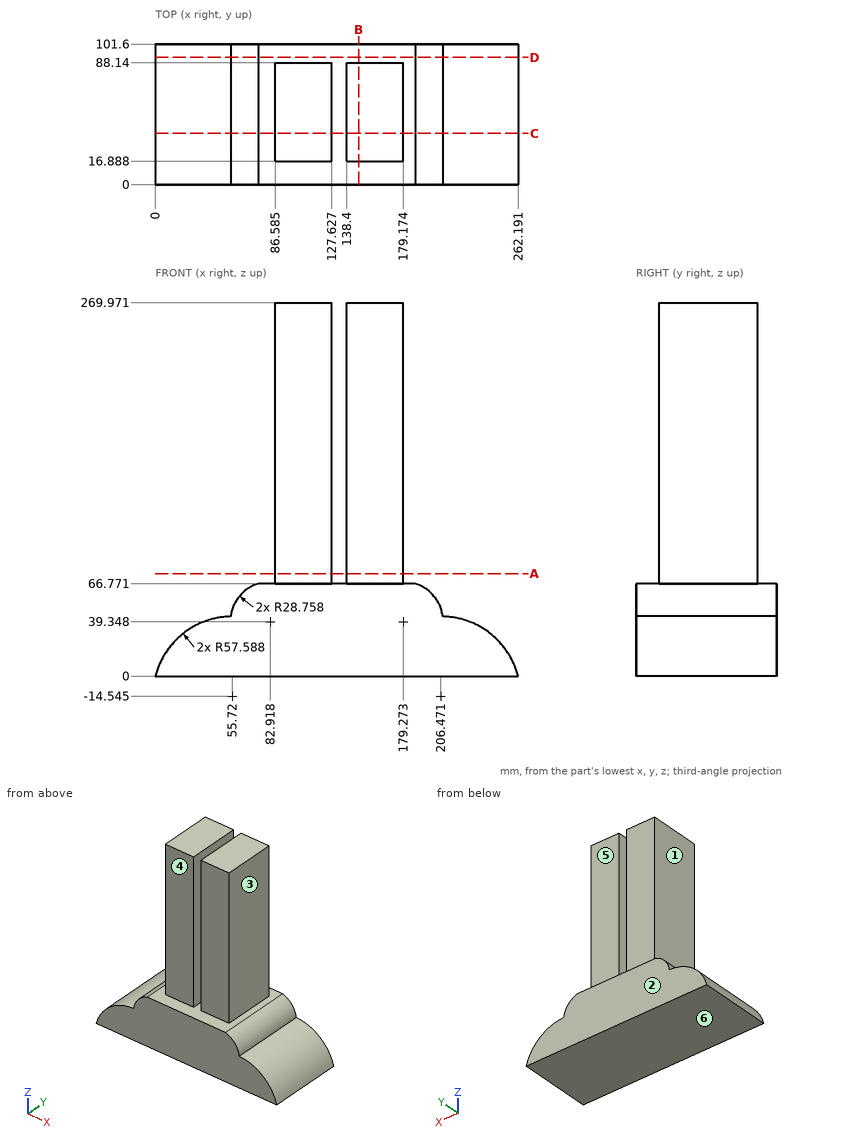
Can you work these out from the drawing? Everything is in mm from the part's minimum corner. A direction names the side the tool comes from. Round coordinates to 2 decimals unless told otherwise and drop trailing zeros. Order: outer loops, then holes, each group sorted by start corner. A loop starts at its lowest first (then second) coordinate and runs counter-clockwise, first axis right, second up. Notation, with made-up numbers: (86, 6.5) -> (90, 6.5) arc R26 ccw to (90, 23.5) -> close; hole circle Ø8 at (35, 61.25). An arc over 180 degrees is marked (long way). Return JSON: item names as keys, results as strings. Group by question number.
1. I need wall thicknesses on line 1 (X direction, y = 69.5, z = 117) (1 decimal); line 2 (Z direction, x = 136, y = 17); line 3 (Y direction, x = 105.5, z = 85). Which ranges of each line are inside material? Lowest first, please. Write a range as [from, to].
2. If we section it at C-C, the plane y = 37: Write out the boundary of the cut face in (x, z) (1 decimal).
3. We'd pull the mould along X, two halves only. Please class the marked faces 1, 2 and 3: released by +X, released by -X, zero draft, split by the parting line, or undercut.
4. If we section it at D-D, the plane y = 92: Write out the boundary of the cut face in (x, z) (1 decimal).
5. Which directions (+Z, -Z, +X, -X, +Y, -Y) give clear straight access to the entire face, cutting with the end or side of a thin tool? Please do the marked faces 4, 5 and 6.
6. If we section it at B-B, the plane x = 147: Write out the boundary of the cut face in (y, z), then the cut area to 3 significant figures.
7. Will these pins go through, and if not, where does the flat tip stop? pin 1 (3 mm diameter, centred on y = 48.5, z = 236, fed in from -X) (1 decimal); pin 2 (3 mm diameter, centred on y = 20, z = 116.5, fed in from +X); pin 3 (4 mm diameter, centred on y = 31.5, z = 31.5, fed in from -X).
8. If we section it at A-A, the plane z = 74: Write out the boundary of the cut face in (x, y) (1 decimal).
Output values:
{
 "1": {"line 1": "[86.6, 127.6], [138.4, 179.2]", "line 2": "[0, 66.77]", "line 3": "[16.89, 88.14]"},
 "2": {"outline": "(0, 0) -> (262.2, 0) arc R57.6 ccw to (207.8, 43) arc R28.8 ccw to (187.9, 66.8) -> (179.2, 66.8) -> (179.2, 270) -> (138.4, 270) -> (138.4, 66.8) -> (127.6, 66.8) -> (127.6, 270) -> (86.6, 270) -> (86.6, 66.8) -> (74.3, 66.8) arc R28.8 ccw to (54.4, 43) arc R57.6 ccw to start"},
 "3": {"face 1": "released by -X", "face 2": "zero draft", "face 3": "released by +X"},
 "4": {"outline": "(0, 0) -> (262.2, 0) arc R57.6 ccw to (207.8, 43) arc R28.8 ccw to (187.9, 66.8) -> (74.3, 66.8) arc R28.8 ccw to (54.4, 43) arc R57.6 ccw to start"},
 "5": {"face 4": "+Z, +X, -X, -Y", "face 5": "+Z, +X, -X, +Y", "face 6": "-Z, +X, -X, +Y, -Y"},
 "6": {"outline": "(0, 0) -> (101.6, 0) -> (101.6, 66.77) -> (88.14, 66.77) -> (88.14, 269.97) -> (16.89, 269.97) -> (16.89, 66.77) -> (0, 66.77) -> close", "area": "21,300 mm²"},
 "7": {"pin 1": "x = 86.6", "pin 2": "x = 179.17", "pin 3": "x = 18.62"},
 "8": {"outline": "(86.6, 16.9) -> (127.6, 16.9) -> (127.6, 88.1) -> (86.6, 88.1) -> close; (138.4, 16.9) -> (179.2, 16.9) -> (179.2, 88.1) -> (138.4, 88.1) -> close"}
}
